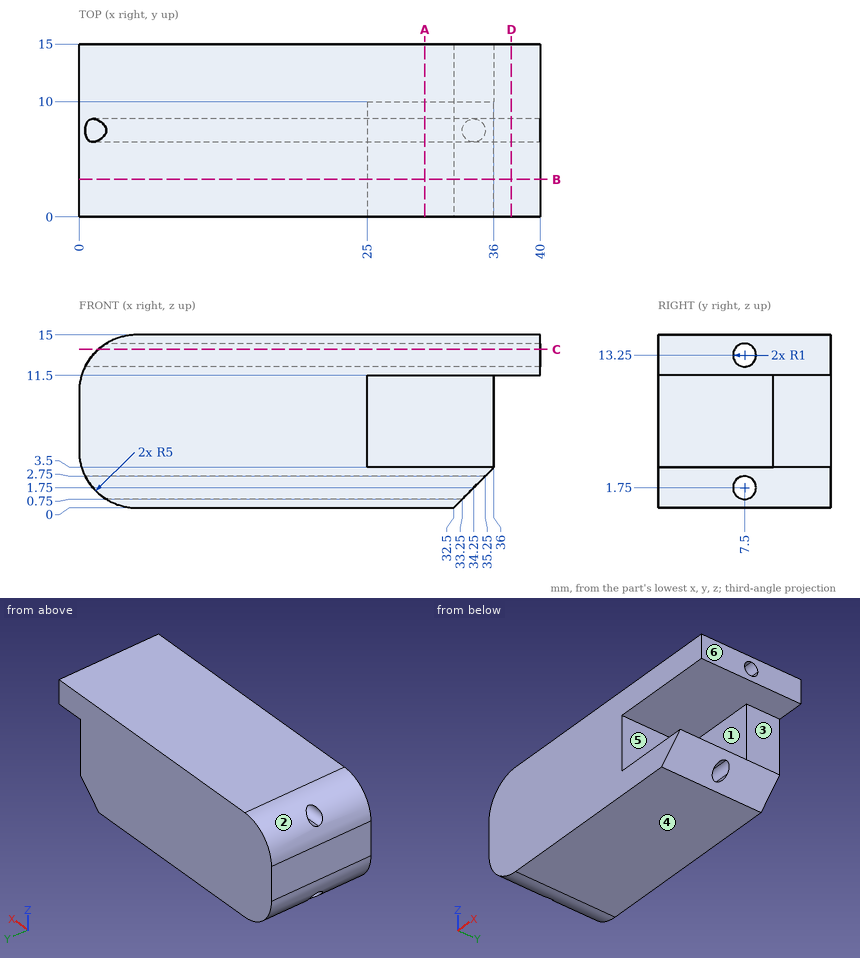
For this review, use the dimensioned drawing (mm, ordinates from the lowest corner) and the shaded views. A direction names the side the tool comes from. Round coordinates to 2 decimals unless told otherwise and drop trailing zeros. Loops run counter-clockwise (first coordinate to the right, second up) from the corner with the lowest first, then second, coordinate; pieces in that order, holes last. Notation, with made-up numbers: (56.25, -10) -> (103.25, -10) arc R27 ccw to (103.25, 24) -> close; hole circle Ø11 at (-8, 29.25). An arc over 180 degrees is marked (long way). Write item = value, one per line. Start each with the question number.
Item 1: For the marked faces 1, 2 and 3, list the 3-axis set-ups (+Z, -Z, +X, -X, +Y, -Y) from which the entire face can be reached by the end or side of a thin tool; tool diameter is ignored.
Item 2: Take a section at C-C on z = 13.75. Give the boundary of the cut face in (x, y), plus the area to 3 significant figures.
Item 3: Take a section at A-A on x = 30. Give the boundary of the cut face in (y, z), plus the area to 3 significant figures.
Item 4: To check wall thickness, follow L1, parallel to Z at x = 30, y = 5.25; L2, parallel to Z at x = 12.5, y = 7.25; L3, parallel to Y at x = 35, z = 10.5. State the ranges of each line that lie inside material, in increasing order.
Item 5: Take a section at B-B on y = 3.25. Give the boundary of the cut face in (x, z), plus the area to 3 significant figures.
Item 6: Mouldability with a two-part tool opening along Z and no side actions: class the marked faces 4, 5 and 6 as released by +Z, released by -Z, zero draft, split by the parting line, or undercut.
Item 7: Take a section at D-D on x = 37.5. Give the boundary of the cut face in (y, z).
Item 8: Insertion check: pin 1 (2.5 mm diameter, centred on x = 28, z = 7, fed in from -Y); pin 2 (6.5 mm diameter, centred on y = 5.5, z = 7.5, fed in from +X); pin 3 (1.5 mm diameter, centred on y = 13.5, z = 7, fed in from +X). Each pin has a flat end and moves straight along its axis. Give the tip position at first contact, or say it passes through.
Result:
q1.face_1 = +X, -Y
q1.face_2 = +Z, -X, +Y, -Y
q1.face_3 = -Z, +X, +Y, -Y
q2.outline = (1.69, 0) -> (40, 0) -> (40, 6.63) -> (1.69, 6.63) -> close; (1.69, 8.37) -> (40, 8.37) -> (40, 15) -> (1.69, 15) -> close
q2.area = 508 mm²
q3.outline = (0, 0) -> (15, 0) -> (15, 15) -> (0, 15) -> (0, 11.5) -> (10, 11.5) -> (10, 3.5) -> (0, 3.5) -> close; hole circle Ø2 at (7.5, 1.75); hole circle Ø2 at (7.5, 13.25)
q3.area = 139 mm²
q4.L1 = 0 to 3.5, 11.5 to 15
q4.L2 = 0 to 0.78, 2.72 to 12.28, 14.22 to 15
q4.L3 = 10 to 15
q5.outline = (0, 5) arc R5 ccw to (5, 0) -> (32.5, 0) -> (36, 3.5) -> (25, 3.5) -> (25, 11.5) -> (40, 11.5) -> (40, 15) -> (5, 15) arc R5 ccw to (0, 10) -> close
q5.area = 449 mm²
q6.face_4 = released by -Z
q6.face_5 = undercut
q6.face_6 = zero draft
q7.outline = (0, 11.5) -> (15, 11.5) -> (15, 15) -> (0, 15) -> close; hole circle Ø2 at (7.5, 13.25)
q8.pin_1 = 10
q8.pin_2 = 25
q8.pin_3 = 36
